Here's how the part is built. I have some questions about the finished solid (model axes, mm). A direction names the side the tool comes from. Coordinates: 2 decimals unless noted, no trailing zeros. Write each loop counter-clockwise with the first axis right and the second up, starting at its lowest first coordinate (ties: lowest second). Pieces come first, ordered by that corner, then holes.
Item 1: We'd pull the mould along X, two halves only. Please class faces 1 (the face through (-12.046, 0.57, 5.568)), 2 (the face through (15.25, 0.57, 5.57)), 3 (the face through (1, 3, 12.159)), 4 (the face through (-9.647, 7, 6)): +X half, -X half, draft (parallel to the pull), parting line (faces both ways), or undercut.
Item 2: For faces 5 (the face through (1, 4, 6)), 6 (the face through (1.2, -5.5, 1.7)), 7 (the face through (-12.647, 6, 6)), which set-ups out of +Z, -Z, +X, -X, +Y, -Y let a thin tool reach every point of the face, with its end or its side?
Item 3: If we section it at C-C (x = 8.5): Please give me the cut outline in (y, z), then the cut area to 3 significant figures.
Item 4: I'm going to push flat-ended pins straight in: pin 1 Ø5 at (x, z) = (8, 3.5) entering from +Y; pin 2 Ø5 at (y, z) = (8.85, 5.66) entering from -X; pin 3 Ø4 at (x, z) = (-5, 9) entering from -Y; pin 4 Ø1.5 at (x, y) = (1.5, -4.5) entering from +Z. Where does each tip first touch, or does it pass through?
Item 5: If I drill on line 1 (X direction, y = 6, z = 7.25); line 2 (Y direction, x = 2.75, z = 5); line 3 (Y direction, x = 2, z = 7.75), over which ranges is the centre line in solid material (lowest first)?
Item 6: If we section it at D-D (z = 4.75): Count the separate pieces of the cut face and the enclosed holes in it, then the cut area to 3 significant figures.
Item 7: If we section it at B-B (z = 9): Please give me the cut outline in (x, y).
Item 8: If we section it at A-A (y = 8.85): Please give me the cut outline in (x, z).
from build123d import *

# Parameters (mm, degrees)
SKETCH1_W           = 28.5
SKETCH1_H           = 17
BOSS_EXTRUDE1_DEPTH = 4
SKETCH2_W           = 3
SKETCH2_H           = 17
BOSS_EXTRUDE2_DEPTH = 8
SKETCH3_R           = 1.5
CUT_EXTRUDE1_DEPTH  = 29.5
SKETCH4_R           = 2
BOSS_EXTRUDE3_DEPTH = 9
FILLET1_R           = 2
FILLET2_R           = 2
FILLET3_R           = 1
SKETCH5_W           = 36.717008867
SKETCH5_H           = 6.82374105
CUT_EXTRUDE2_DEPTH  = 12


with BuildPart() as part:
    # Sketch1 → Boss-Extrude1 (new body)
    with BuildSketch(Plane(origin=(0, 0, 0), x_dir=(1, 0, 0), z_dir=(0, 1, 0))):
        with Locations((1.602817149, -3.658837531)):
            Rectangle(SKETCH1_W, SKETCH1_H)
    extrude(amount=BOSS_EXTRUDE1_DEPTH)

    # Sketch2 → Boss-Extrude2 (add)
    with BuildSketch(Plane(origin=(0, 4, 0), x_dir=(1, 0, 0), z_dir=(0, 1, 0))):
        with Locations((-11.147182851, -3.658837531)):
            Rectangle(SKETCH2_W, SKETCH2_H)
        with Locations((14.352817149, -3.658837531)):
            Rectangle(SKETCH2_W, SKETCH2_H)
    extrude(amount=BOSS_EXTRUDE2_DEPTH)

    # Sketch3 → Cut-Extrude1 (cut, through all)
    with BuildSketch(Plane.ZY.offset(12.647182851)):
        with Locations((5.658837531, 8.85)):
            Circle(SKETCH3_R)
    extrude(amount=-CUT_EXTRUDE1_DEPTH, mode=Mode.SUBTRACT)

    # Sketch4 → Boss-Extrude3 (add)
    with BuildSketch(Plane.XZ):
        with Locations((1.602817149, 3.658837531)):
            Circle(SKETCH4_R)
    extrude(amount=BOSS_EXTRUDE3_DEPTH)

    # Fillet1
    fillet1_edges = [part.edges().sort_by_distance(p)[0] for p in [
        (-0.397182851, 0, 3.658837531),
    ]]
    fillet(fillet1_edges, radius=FILLET1_R)

    # Fillet2
    fillet2_edges = [part.edges().sort_by_distance(p)[0] for p in [
        (15.852817149, 0, 3.658837531),
        (-12.647182851, 0, 3.658837531),
    ]]
    fillet(fillet2_edges, radius=FILLET2_R)

    # Fillet3
    fillet3_edges = [part.edges().sort_by_distance(p)[0] for p in [
        (-12.647182851, 12, 3.658837531),
        (-9.647182851, 12, 3.658837531),
        (15.852817149, 12, 3.658837531),
        (12.852817149, 12, 3.658837531),
    ]]
    fillet(fillet3_edges, radius=FILLET3_R)

    # Sketch5 → Cut-Extrude2 (cut)
    with BuildSketch(Plane.XZ):
        with Locations((1.100738545, -4.253032994)):
            Rectangle(SKETCH5_W, SKETCH5_H)
    extrude(amount=-CUT_EXTRUDE2_DEPTH, mode=Mode.SUBTRACT)


solid = part.part
Answer list:
1. face 1: -X half
1. face 2: +X half
1. face 3: draft
1. face 4: undercut
2. face 5: +Z, -Z, +Y
2. face 6: -Y
2. face 7: +Z, -Z, -X, +Y, -Y
3. outline: (0, -0.84) - (4, -0.84) - (4, 12.16) - (0, 12.16) - close
3. area: 52.0 mm2
4. pin 1: stops at y = 4
4. pin 2: stops at x = -12.65
4. pin 3: stops at y = 0
4. pin 4: stops at z = 5.66
5. line 1: x = -12.65 to -9.65, 12.85 to 15.85
5. line 2: y = -9 to 4
5. line 3: y = 0 to 4
6. separate pieces: 3
6. enclosed holes: 0
6. area: 177 mm2
7. outline: (-12.65, 2) arc R2 ccw to (-10.65, 0) - (13.85, 0) arc R2 ccw to (15.85, 2) - (15.85, 11) arc R1 ccw to (14.85, 12) - (13.85, 12) arc R1 ccw to (12.85, 11) - (12.85, 4) - (-9.65, 4) - (-9.65, 11) arc R1 ccw to (-10.65, 12) - (-11.65, 12) arc R1 ccw to (-12.65, 11) - close
8. outline: (-12.65, -0.84) - (-9.65, -0.84) - (-9.65, 4.16) - (-12.65, 4.16) - close; (-12.65, 7.16) - (-9.65, 7.16) - (-9.65, 12.16) - (-12.65, 12.16) - close; (12.85, -0.84) - (15.85, -0.84) - (15.85, 4.16) - (12.85, 4.16) - close; (12.85, 7.16) - (15.85, 7.16) - (15.85, 12.16) - (12.85, 12.16) - close
